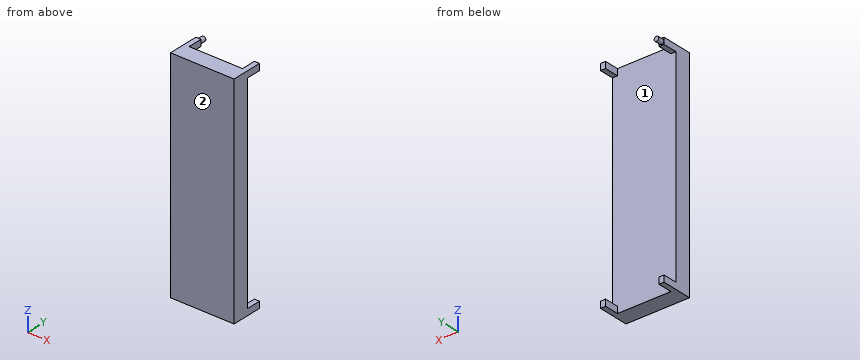
from build123d import *

# Parameters (mm, degrees)
SKETCH1_W           = 97.663
SKETCH1_H           = 336.55
BASE_DEPTH          = 25.4
SKETCH2_W           = 7.874
SKETCH2_H           = 9.906
BOSS_EXTRUDE2_DEPTH = 22.225
SKETCH3_R           = 3.556
BOSS_EXTRUDE3_DEPTH = 9.398


with BuildPart() as part:
    # Sketch1 → Base (new body)
    with BuildSketch(Plane(origin=(0, 0, 0), x_dir=(1, 0, 0), z_dir=(0, 1, 0))):
        Rectangle(SKETCH1_W, SKETCH1_H)
    extrude(amount=BASE_DEPTH)

    # Sketch2 → Boss-Extrude2 (add)
    with BuildSketch(Plane(origin=(0, 25.4, 0), x_dir=(1, 0, 0), z_dir=(0, 1, 0))):
        with Locations((-44.8945, -163.322)):
            Rectangle(SKETCH2_W, SKETCH2_H)
        with Locations((44.8945, -163.322)):
            Rectangle(SKETCH2_W, SKETCH2_H)
        with Locations((44.8945, 163.322)):
            Rectangle(SKETCH2_W, SKETCH2_H)
        with Locations((-44.8945, 163.322)):
            Rectangle(SKETCH2_W, SKETCH2_H)
    extrude(amount=BOSS_EXTRUDE2_DEPTH)

    # Sketch3 → Boss-Extrude3 (add)
    with BuildSketch(Plane(origin=(0, 47.625, 0), x_dir=(1, 0, 0), z_dir=(0, 1, 0))):
        with Locations(Location((-44.8945, -163.322, 0), (0, 0, 90))):
            Circle(SKETCH3_R)
    extrude(amount=BOSS_EXTRUDE3_DEPTH)


solid = part.part
Read the model definition and answer for the solid it produces. Units are mm, in the model's axes. Face numbers are marked on the shaded views. Coordinates: 2 decimals unless noted, no trailing zeros. Order: outer loops, then holes, each group sorted by start corner. A loop starts at its lowest first (then second) coordinate and runs counter-clockwise, first axis right, second up. Notation, with made-up numbers: (60, 85) - (97, 85) arc R22 ccw to (97, 107) - close; hole circle Ø2 at (24, -13). An arc over 180 degrees is marked (long way). Use one line per item in the form item = value.
(1) Section A-A, the plane y = 34.5 is taken. Give the vertices of the cut face in (x, z) (1 decimal).
Computed values:
outline = (-48.8, -168.3) - (-41, -168.3) - (-41, -158.4) - (-48.8, -158.4) - close; (-48.8, 158.4) - (-41, 158.4) - (-41, 168.3) - (-48.8, 168.3) - close; (41, -168.3) - (48.8, -168.3) - (48.8, -158.4) - (41, -158.4) - close; (41, 158.4) - (48.8, 158.4) - (48.8, 168.3) - (41, 168.3) - close
(2) Section B-B, the plane z = 61 is taken. Give the vertices of the cut face in (x, y).
Computed values:
outline = (-48.83, 0) - (48.83, 0) - (48.83, 25.4) - (-48.83, 25.4) - close
(3) For a pull along Z with two mould halves and no side action, classify the marked faces 1 and 2 as pulls with the +Z half, pulls with the -Z half, needs draft (parallel to the pull), parting line crosses it, or undercut.
Computed values:
face_1 = undercut
face_2 = needs draft
(4) Given pin 1 Ø6 at (x, z) = (18, 78.5) entering from -Y; pin 2 Ø6.5 at (x, z) = (43, -161) entering from +Y (3 decimals), each flat-ended and moving along its own axis, determine where each tip first touches the part or whether it passes through.
Computed values:
pin_1 = 0
pin_2 = 47.625
(5) Section C-C, the plane x = 33.5 is taken. Give the vertices of the cut face in (y, z) (3 decimals), then the cut area to 3 significant figures.
Computed values:
outline = (0, -168.275) - (25.4, -168.275) - (25.4, 168.275) - (0, 168.275) - close
area = 8,550 mm²
(6) A straight line is drawn through the part: L1, parallel to Y at x = 26, z = -138. Find the intervals that lie inside material, in ascending order.
Computed values:
L1 = 0 to 25.4
